The listing builds one solid part. Answer for the finished solid, in the listing's coordinates (mm). Coordinates: 2 decimals unless noted, no trailing zeros. Order: outer loops, then holes, each group sorted by start corner. A loop starts at its lowest first (then second) coordinate and runs counter-clockwise, first axis right, second up. Notation, with made-up numbers: (83.25, 12) - (137.25, 12) arc R23 ccw to (137.25, 40) - close; hole circle Ø5 at (17, 63). An arc over 180 degrees is marked (long way). One line per item, written item: value. Start each with the question number.
```python
from build123d import *

# Parameters (mm, degrees)
EXTRUDE_1_DEPTH     = 3
SKETCH_1_3_R        = 2.25
CUT_EXTRUDE_1_DEPTH = 1.5
SKETCH_1_4_R        = 1.5
CUT_EXTRUDE_2_DEPTH = 3


with BuildPart() as part:
    # 草图1 → 凸台-拉伸1 (new body)
    with BuildSketch(Plane.XY):
        with BuildLine():
            Line((-68, 39.2), (295.5, 39.2))
            ThreePointArc((295.5, 39.2), (302.571067812, 36.271067812), (305.5, 29.2))
            Line((305.5, 29.2), (305.5, -240))
            ThreePointArc((305.5, -240), (302.571067812, -247.071067812), (295.5, -250))
            Line((295.5, -250), (-68, -250))
            ThreePointArc((-68, -250), (-75.071067812, -247.071067812), (-78, -240))
            Line((-78, -240), (-78, 29.2))
            ThreePointArc((-78, 29.2), (-75.071067812, 36.271067812), (-68, 39.2))
        make_face()
    extrude(amount=EXTRUDE_1_DEPTH)

    # 草图1<3> → 切除-拉伸1 (cut)
    with BuildSketch(Plane.XY):
        with Locations((6.75, -12.5)):
            Circle(SKETCH_1_3_R)
        with Locations((140.25, -12.5)):
            Circle(SKETCH_1_3_R)
        with Locations((140.25, -231)):
            Circle(SKETCH_1_3_R)
        with Locations((6.75, -231)):
            Circle(SKETCH_1_3_R)
        with Locations((155.25, -12.5)):
            Circle(SKETCH_1_3_R)
        with Locations((288.75, -12.5)):
            Circle(SKETCH_1_3_R)
        with Locations((288.75, -231)):
            Circle(SKETCH_1_3_R)
        with Locations((155.25, -231)):
            Circle(SKETCH_1_3_R)
    extrude(amount=CUT_EXTRUDE_1_DEPTH, mode=Mode.SUBTRACT)

    # 草图1<4> → 切除-拉伸2 (cut)
    with BuildSketch(Plane.XY):
        with Locations((6.75, -12.5)):
            Circle(SKETCH_1_4_R)
        with Locations((140.25, -12.5)):
            Circle(SKETCH_1_4_R)
        with Locations((140.25, -231)):
            Circle(SKETCH_1_4_R)
        with Locations((6.75, -231)):
            Circle(SKETCH_1_4_R)
        with Locations((155.25, -12.5)):
            Circle(SKETCH_1_4_R)
        with Locations((288.75, -12.5)):
            Circle(SKETCH_1_4_R)
        with Locations((288.75, -231)):
            Circle(SKETCH_1_4_R)
        with Locations((155.25, -231)):
            Circle(SKETCH_1_4_R)
        with BuildLine():
            Line((31.5, -60), (115.5, -60))
            ThreePointArc((115.5, -60), (117.621320344, -60.878679656), (118.5, -63))
            Line((118.5, -63), (118.5, -177))
            ThreePointArc((118.5, -177), (117.621320344, -179.121320344), (115.5, -180))
            Line((115.5, -180), (31.5, -180))
            ThreePointArc((31.5, -180), (29.378679656, -179.121320344), (28.5, -177))
            Line((28.5, -177), (28.5, -63))
            ThreePointArc((28.5, -63), (29.378679656, -60.878679656), (31.5, -60))
        make_face()
        with BuildLine():
            Line((180, -60), (264, -60))
            ThreePointArc((264, -60), (266.121320344, -60.878679656), (267, -63))
            Line((267, -63), (267, -177))
            ThreePointArc((267, -177), (266.121320344, -179.121320344), (264, -180))
            Line((264, -180), (180, -180))
            ThreePointArc((180, -180), (177.878679656, -179.121320344), (177, -177))
            Line((177, -177), (177, -63))
            ThreePointArc((177, -63), (177.878679656, -60.878679656), (180, -60))
        make_face()
    extrude(amount=CUT_EXTRUDE_2_DEPTH, mode=Mode.SUBTRACT)


solid = part.part
```
(1) The part is cut by section A-A on x = 255.5. Determine the outline of the cut face in (y, z).
(2) Consider probe 1 along X at (y, z) = (-101.5, 0.65); probe 2 along Y at (x, z) = (140.25, 2.55); probe 3 along Y at (x, z) = (288.75, 0.8). Determine where each line is inside the solid, lowest interval first.
(3) The part is cut by section B-B on y = -92.5. Determine the outline of the cut face in (x, z), plus the area to 4 significant figures.
(4) The part is cut by section C-C on z = 2.5. Count the separate pieces of the cut face and the enclosed holes in it, plus the area to 3 significant figures.
(5) Flat-ended cylindrical pins translate along their axes: pin 1 Ø3.5 at (x, y) = (288.75, -231) entering from -Z; pin 2 Ø5 at (x, y) = (6.75, -231) entering from -Z. Find the tip coordinate at first contact, or state that the pin passes through.
Completed:
1. outline: (-250, 0) - (-180, 0) - (-180, 3) - (-250, 3) - close; (-60, 0) - (39.2, 0) - (39.2, 3) - (-60, 3) - close
2. probe 1: x = -78 to 28.5, 118.5 to 177, 267 to 305.5
2. probe 2: y = -250 to -232.5, -229.5 to -14, -11 to 39.2
2. probe 3: y = -250 to -233.25, -228.75 to -14.75, -10.25 to 39.2
3. outline: (-78, 0) - (28.5, 0) - (28.5, 3) - (-78, 3) - close; (118.5, 0) - (177, 0) - (177, 3) - (118.5, 3) - close; (267, 0) - (305.5, 0) - (305.5, 3) - (267, 3) - close
3. area: 610.5 mm2
4. separate pieces: 1
4. enclosed holes: 10
4. area: 89,200 mm2
5. pin 1: stops at z = 1.5
5. pin 2: stops at z = 0
